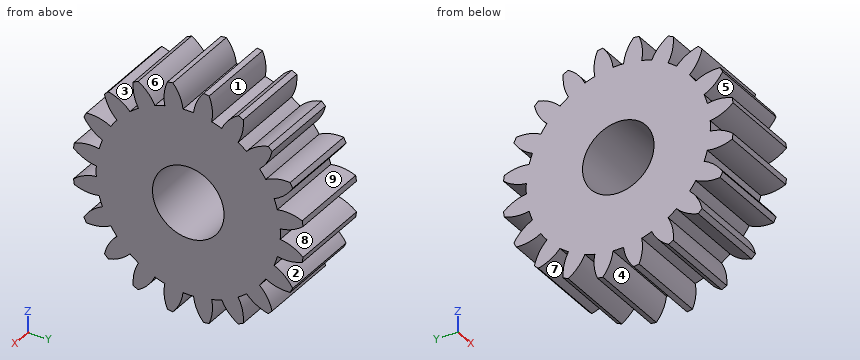
```python
from build123d import *

# Parameters (mm, degrees)
BASPROSKE_W         = 10
BASPROSKE_H         = 13.75
TOOTHCUT_DEPTH      = 22.866069606
TEETHCUTS_COUNT     = 20
TEETHCUTS_ANGLE     = 342
BORSKE_R            = 2
BORE_DEPTH          = 50.0000508
SKETCH2_R           = 2
BOSS_EXTRUDE1_DEPTH = 10
SKETCH3_R           = 4.25
CUT_EXTRUDE2_DEPTH  = 10


with BuildPart() as part:
    # BasProSke → Base-Revolve (revolve)
    with BuildSketch(Plane(origin=(0, 0, 0), x_dir=(1, 0, 0), z_dir=(0, 1, 0)), mode=Mode.PRIVATE) as base_revolve_sk:
        with Locations((5, 6.875)):
            Rectangle(BASPROSKE_W, BASPROSKE_H)
    revolve(base_revolve_sk.sketch.rotate(Axis((-10, 0, 0), (1, 0, 0)), 180), axis=Axis((-10, 0, 0), (1, 0, 0)))

    # TooCutSke → ToothCut (cut, through all)
    with BuildSketch(Plane(origin=(0, 0, 0), x_dir=(0, 0, -1), z_dir=(1, 0, 0))):
        with BuildLine():
            ThreePointArc((0.62110296, 10.918848994), (0, 10.9365), (-0.62110296, 10.918848994))
            ThreePointArc((-0.62110296, 10.918848994), (-1.024517052, 12.378857135), (-1.846615859, 13.651067908))
            ThreePointArc((-1.846615859, 13.651067908), (0, 13.7754), (1.846615859, 13.651067908))
            ThreePointArc((1.846615859, 13.651067908), (1.024517052, 12.378857135), (0.62110296, 10.918848994))
        make_face()
    toothcut = extrude(amount=TOOTHCUT_DEPTH, mode=Mode.SUBTRACT)

    # TeethCuts: ToothCut ×20 about axis
    teethcuts_axis = Axis((-10, 0, 0), (1, 0, 0))
    for i in range(1, TEETHCUTS_COUNT):
        add(toothcut.rotate(teethcuts_axis, i * TEETHCUTS_ANGLE / (TEETHCUTS_COUNT - 1)), mode=Mode.SUBTRACT)

    # BorSke → Bore (cut, symmetric)
    with BuildSketch(Plane(origin=(0, 0, 0), x_dir=(0, 0, -1), z_dir=(1, 0, 0))):
        with Locations(Location((0, 0, 0), (0, 0, 180))):
            Circle(BORSKE_R)
    extrude(amount=BORE_DEPTH, both=True, mode=Mode.SUBTRACT)

    # Sketch2 → Boss-Extrude1 (add)
    with BuildSketch(Plane(origin=(10, 0, 0), x_dir=(0, 0, -1), z_dir=(1, 0, 0))):
        Circle(SKETCH2_R)
    extrude(amount=-BOSS_EXTRUDE1_DEPTH)

    # Sketch3 → Cut-Extrude2 (cut)
    with BuildSketch(Plane(origin=(10, 0, 0), x_dir=(0, 0, -1), z_dir=(1, 0, 0))):
        Circle(SKETCH3_R)
    extrude(amount=-CUT_EXTRUDE2_DEPTH, mode=Mode.SUBTRACT)


solid = part.part
```
Geometry check sheet. Reference: the model listing, model coordinates, mm. Face numbers are marked on the shaded views. A direction names the side the tool comes from. Give positions to 0.01 mm unless a question says otherwise; leave off trailing zeros. Loops run counter-clockwise (first coordinate to the right, second up) from the corner with the lowest first, then second, coordinate; pieces in that order, holes last. Notation, with made-up numbers: (55.5, 51) - (61.5, 51) arc R25 ccw to (61.5, 67) - close; hole circle Ø5 at (2, 48). An arc over 180 degrees is marked (long way). Use CSV: the item, a comma, the result in double quotes. Start each with the question number.
Q1. Section check C-C, the plane z = 7.5. Record the cut outline in (x, y).
Q2. Release check for a two-part mould opening along Z. For the marked faces 6, 7, 8 and 9 record: +Z half, -Z half, draft (parallel to the pull), parting line (faces both ways), or undercut.
Q3. Scan lines: probe 1 along Z at (x, y) = (1.5, 8.75); probe 2 along Y at (x, z) = (0.5, -11.75); probe 3 along Z at (x, y) = (0.75, -11.5). Record each from-to range of solid material in increasing order. Write a range as from..to.
Q4. Section check A-A, the plane z = 0. Record the cut outline in (x, y).
Q5. Access from +Z, -Z, +X, -X, +Y, -Y to the whole of each face (thin tool, end or side, straight path). Record for the marked faces 1, 2, 3, 4 and 5.
Q6. Go/stop test with flat-tipped pins: pin 1 Ø2 at (x, z) = (7, 8) entering from -Y; pin 2 Ø4 at (x, z) = (3, 5) entering from +Y; pin 3 Ø5 at (y, z) = (0, 0) entering from -X. Record where each tip stops, or that it passes through.
Findings below:
1,outline,"(0, -9) - (10, -9) - (10, 9) - (0, 9) - close"
2,face 6,"+Z half"
2,face 7,"-Z half"
2,face 8,"undercut"
2,face 9,"undercut"
3,probe 1,"z = -9.72..-7.2, -6.56..6.56, 7.2..9.72"
3,probe 2,"y = -6.55..-5.09, -2.88..-0.79, 0.79..2.88, 5.09..6.55"
3,probe 3,"z = -6.55..-4.84, -2.88..-0.72, 0.72..2.88, 4.84..6.55"
4,outline,"(0, -10.94) - (10, -10.94) - (10, -4.25) - (0, -4.25) - close; (0, 4.25) - (10, 4.25) - (10, 10.94) - (0, 10.94) - close"
5,face 1,"+X, -X"
5,face 2,"+X, -X, +Y"
5,face 3,"+Z, +X, -X"
5,face 4,"-Z, +X, -X"
5,face 5,"+X, -X, -Y"
6,pin 1,"stops at y = -9.81"
6,pin 2,"stops at y = 12.4"
6,pin 3,"passes through"
